Verification items for the finished model (mm, model axes). Face numbers are marked on the shaded views. A direction names the side the tool comes from. Round coordinates to 2 decimals unless told otherwise and drop trailing zeros. One line per question, with ' | ' between items.
from build123d import *

# Parameters (mm, degrees)
F0_R     = 68.2625
F0_R_2   = 27.0256
F1_DEPTH = 69.85
F3_R     = 31.75
F4_DEPTH = 19.05
F5_W     = 12.7
F5_H     = 33.3375
F6_DEPTH = 69.851
F7_SIZE  = 1.27
F8_D     = 10.71626
F8_DEPTH = 63.5
F8_TIP   = 3.2194893086


with BuildPart() as f1:
    # F0 (on Top) → F1 (new body)
    with BuildSketch(Plane.XY):
        Circle(F0_R)
        Circle(F0_R_2, mode=Mode.SUBTRACT)
    extrude(amount=F1_DEPTH)

    # F3 (on face) → F4 (cut)
    with BuildSketch(Plane(origin=(0, 0, 0), x_dir=(1, 0, 0), z_dir=(0, 0, -1))):
        Circle(F3_R)
    extrude(amount=-F4_DEPTH, mode=Mode.SUBTRACT)

    # F5 (on face) → F6 (cut, through all)
    with BuildSketch(Plane(origin=(0, 0, 0), x_dir=(1, 0, 0), z_dir=(0, 0, -1))):
        with Locations((0, 16.66875)):
            Rectangle(F5_W, F5_H)
    extrude(amount=-F6_DEPTH, mode=Mode.SUBTRACT)

    # F7
    f7_edges = [f1.edges().sort_by_distance(p)[0] for p in [
        (-68.2625, 0, 69.85),
        (-68.2625, 0, 0),
    ]]
    chamfer(f7_edges, length=F7_SIZE)

    # F8
    with Locations(Plane(origin=(0, 0, 0), x_dir=(1, 0, 0), z_dir=(0, 0, -1))):
        with Locations((0, 57.15), (-49.4933518263, 28.575), (49.4933518263, 28.575), (49.4933518263, -28.575), (0, -57.15), (-49.4933518263, -28.575)):
            Hole(F8_D / 2, depth=F8_DEPTH)
            with Locations((0, 0, -(F8_DEPTH + F8_TIP / 2))):  # 118° drill point
                Cone(0, F8_D / 2, F8_TIP, mode=Mode.SUBTRACT)


solid = f1.part
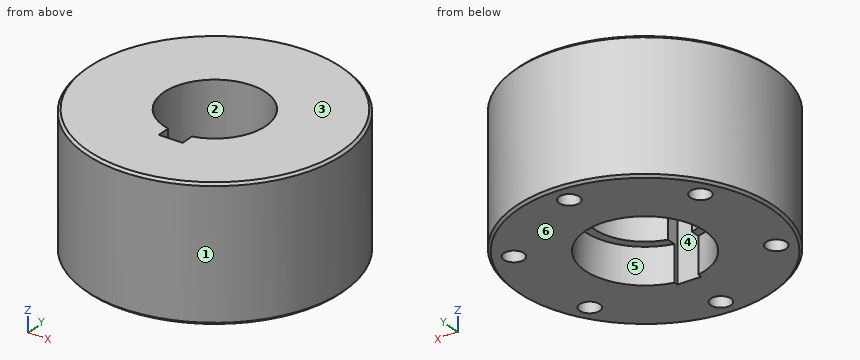
1. Go/stop test with flat-tipped pins: P1, Ø6, axis at y = -23, z = 20.5, coming from the -X side; P2, Ø4, axis at x = -48, z = 31.5, coming from the +Y side; P3, Ø14, axis at x = 1, z = 24, coming from the +Y side. Record where each tip stops, or that it passes through.
Results:
P1: stops at x = -65.27 | P2: stops at y = 50.44 | P3: stops at y = 68.26
2. Thickness scan on line 1 (X direction, y = -29.5, z = 56.5); line 2 (Y direction, x = -52.5, z = 15); line 3 (Y direction, x = 0, z = 44). Record the ranges inside material, lowest first.
Results:
line 1: x = -61.56 to -54.77, -44.22 to -6.35, 6.35 to 44.22, 54.77 to 61.56 | line 2: y = -43.63 to -33.01, -24.14 to 24.14, 33.01 to 43.63 | line 3: y = -68.26 to -62.51, -51.79 to -33.34, 27.03 to 51.79, 62.51 to 68.26
3. Mould release check, pull along X, two halves, no side actions. Record for the marked faces 1, 2 and 3: pulls with the +X half, pulls with the -X half, needs draft (parallel to the pull), parting line crosses it, or undercut.
Results:
face 1: parting line crosses it | face 2: undercut | face 3: needs draft
4. Tool access check on the marked faces 4, 5 and 6. Record the directions out of +Z, -Z, +X, -X, +Y, -Y that give a thin tool (end or side, any length) a straight path to the whole face; none if there is none.
Results:
face 4: +Z, -Z | face 5: -Z | face 6: -Z, +X, -X, +Y, -Y
5. Section check A-A, the plane z = 27.5. Count the separate pieces of the cut face and the enclosed holes in it, then the cut area to 3 significant figures.
Results:
separate pieces: 1 | enclosed holes: 7 | area: 11,700 mm2
